from build123d import *

# Parameters (mm, degrees)
SKETCH1_R           = 3.175
BOSS_EXTRUDE1_DEPTH = 6.35


with BuildPart() as part:
    # Sketch1 → Boss-Extrude1 (new body)
    with BuildSketch(Plane.XY):
        with BuildLine():
            Line((20.284910643, 0), (20.284910643, 12.632459137))
            add(Edge.make_bspline(
                [(20.284910643, 12.632459137), (11.321554309, 17.627045812), (9.14548831, 30.766646824), (7.127170197, 44.232555484), (5.239939742, 48.001283958)],
                knots=[0, 0, 0, 0, 0.567527293, 0.844926431, 0.844926431, 0.844926431, 0.844926431], degree=3))
            ThreePointArc((5.239939742, 48.001283958), (0, 51.435), (-5.239939742, 48.001283958))
            add(Edge.make_bspline(
                [(-20.284910643, 12.632459137), (-11.321554309, 17.627045812), (-9.14548831, 30.766646824), (-7.127170197, 44.232555484), (-5.239939742, 48.001283958)],
                knots=[0, 0, 0, 0, 0.567527293, 0.844926431, 0.844926431, 0.844926431, 0.844926431], degree=3))
            Line((-20.284910643, 12.632459137), (-20.284910643, 0))
            Line((-20.284910643, 0), (20.284910643, 0))
        make_face()
        with Locations((0, 45.72)):
            Circle(SKETCH1_R, mode=Mode.SUBTRACT)
    extrude(amount=BOSS_EXTRUDE1_DEPTH)


solid = part.part
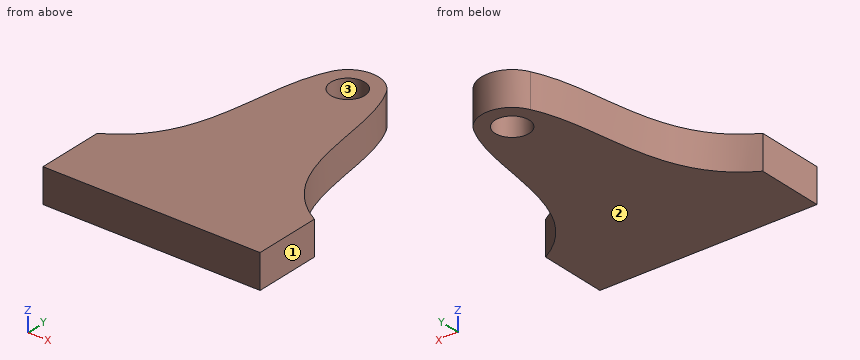
Build history of the part. All positions in model axes, mm. Face numbers are marked on the shaded views. Give positions to 0.01 mm unless a question says otherwise; leave off trailing zeros. Order: outer loops, then holes, each group sorted by start corner. A loop starts at its lowest first (then second) coordinate and runs counter-clockwise, first axis right, second up. Notation, with made-up numbers: M -18.5,48.25 L 24.5,48.25 A8 cw 24.5,54.25 Z; hole C 10.25,53 d3. An arc over 180 degrees is marked long. Put each result on its own line as item: value.
Item 1: Flat gauge pin, fed straight in: pin 1 Ø5.5 at (x, y) = (0, 45.72) entering from -Z. Where does the tip first touch, or does it go through?
From the geometry:
pin 1: passes through
Item 2: Two-plate mould, pull along X, no slides. Class the marked faces 1, 2 and 3: +X half, -X half, draft (parallel to the pull), parting line (faces both ways), or undercut.
From the geometry:
face 1: +X half
face 2: draft
face 3: undercut
Item 3: Slice it at A-A, the plane x = 0. Write the cut outline in (y, z) (3 decimals), plus the area to 3 significant figures.
From the geometry:
outline: M 0,0 L 42.545,0 L 42.545,6.35 L 0,6.35 Z; M 48.895,0 L 51.435,0 L 51.435,6.35 L 48.895,6.35 Z
area: 286 mm2
Item 4: Probe line 1 (Y direction, x = 0, z = 3.25) (3 decimals); line 2 (X direction, y = 45, z = 3.5); line 3 (X direction, y = 30, z = 0.75). List the from-to ranges inside material, lowest first. Write a range as [from, to].
From the geometry:
line 1: y = [0, 42.545], [48.895, 51.435]
line 2: x = [-6.47, -3.09], [3.09, 6.47]
line 3: x = [-9.39, 9.39]
